Input: part model. Units: mm. Frame: model coordinates. A direction names the side the tool comes from. Coordinates: 2 decimals unless noted, no trailing zeros. Loops run counter-clockwise (first coordinate to the right, second up) from the corner with the lowest first, then second, coordinate; pieces in that order, holes last.
Item 1: Contact query for flat-ended pins moving along their axis: P1, Ø1.5, axis at x = -28, z = -1, coming from the +Y side; P2, Ø5, axis at x = -18.5, z = 2, coming from the -Y side; P3, Ø8, axis at x = -66.5, z = 5.5, coming from the +Y side. Output: stop coordinate, or through.
Item 2: Section C-C on z = 6.5. Return loops of the section in (x, y), and give its area (3 significant figures).
Item 3: Ray query, line 1 along Y through (x, z) = (0, 7.75); line 2 along X through (y, z) = (2, -8.25); line 3 along Y through (x, z) = (0, -0.25). Return the intervals inside material, ascending.
Item 4: Pull-direction query (X, two-part tool) for faces 1 (the flat face through (-21, 92, 10.16)), 2 (the flat face through (-69.2, 62.2, 3.175)), 3 (the cylindrical face through (-92.063, -28.992, 0.142)); classes: released by +X, released by -X, zero draft, split by the parting line, or undercut.
Item 5: Reachability of faces 4 (the cylindrical face through (74.579, 57.185, 6.619)), 5 (the cylindrical face through (74.579, 57.185, -6.716)), 6 (the cylindrical face through (-42.428, 81.574, -0.034)) from +Z, -Z, +X, -X, +Y, -Y: full face, straight path, thin tool, end or side. Return the list, or none.
Item 6: Section A-A on x = 0. Return loops of the section in (y, z) (3 decimals), and give its area (3 significant figures).
```python
from build123d import *


with BuildPart() as part:
    # Sketch2 → Revolve1 (revolve)
    with BuildSketch(Plane(origin=(0, 0, 0), x_dir=(0, 0, -1), z_dir=(1, 0, 0)), mode=Mode.PRIVATE) as revolve1_sk:
        with BuildLine():
            Line((-3.175, 93.98), (-3.175, 92.71))
            ThreePointArc((-3.175, 92.71), (-2.951815367, 92.171184633), (-2.413, 91.948))
            Line((-2.413, 91.948), (2.413, 91.948))
            ThreePointArc((2.413, 91.948), (2.951815367, 92.171184633), (3.175, 92.71))
            Line((3.175, 92.71), (3.175, 93.98))
            Line((3.175, 93.98), (10.16, 93.98))
            Line((10.16, 93.98), (10.16, 96.52))
            Line((10.16, 96.52), (-10.16, 96.52))
            Line((-10.16, 96.52), (-10.16, 93.98))
            Line((-10.16, 93.98), (-3.175, 93.98))
        make_face()
    revolve(revolve1_sk.sketch.rotate(Axis((0, 0, -11.176), (0, 0, 1)), 90), axis=Axis((0, 0, -11.176), (0, 0, 1)))


solid = part.part
```
Results found:
1. P1: stops at y = 92.59
1. P2: stops at y = -95.18
1. P3: stops at y = 73.55
2. outline: circle Ø193.04 at (0, 0); hole circle Ø187.96 at (0, 0)
2. area: 1,520 mm2
3. line 1: y = -96.52 to -93.98, 93.98 to 96.52
3. line 2: x = -96.5 to -93.96, 93.96 to 96.5
3. line 3: y = -96.52 to -91.95, 91.95 to 96.52
4. face 1: zero draft
4. face 2: undercut
4. face 3: split by the parting line
5. face 4: +Z
5. face 5: -Z
5. face 6: +Z, -Z
6. outline: (-96.52, -10.16) - (-93.98, -10.16) - (-93.98, -3.175) - (-92.71, -3.175) arc R0.762 ccw to (-91.948, -2.413) - (-91.948, 2.413) arc R0.762 ccw to (-92.71, 3.175) - (-93.98, 3.175) - (-93.98, 10.16) - (-96.52, 10.16) - close; (91.948, -2.413) arc R0.762 ccw to (92.71, -3.175) - (93.98, -3.175) - (93.98, -10.16) - (96.52, -10.16) - (96.52, 10.16) - (93.98, 10.16) - (93.98, 3.175) - (92.71, 3.175) arc R0.762 ccw to (91.948, 2.413) - close
6. area: 129 mm2
